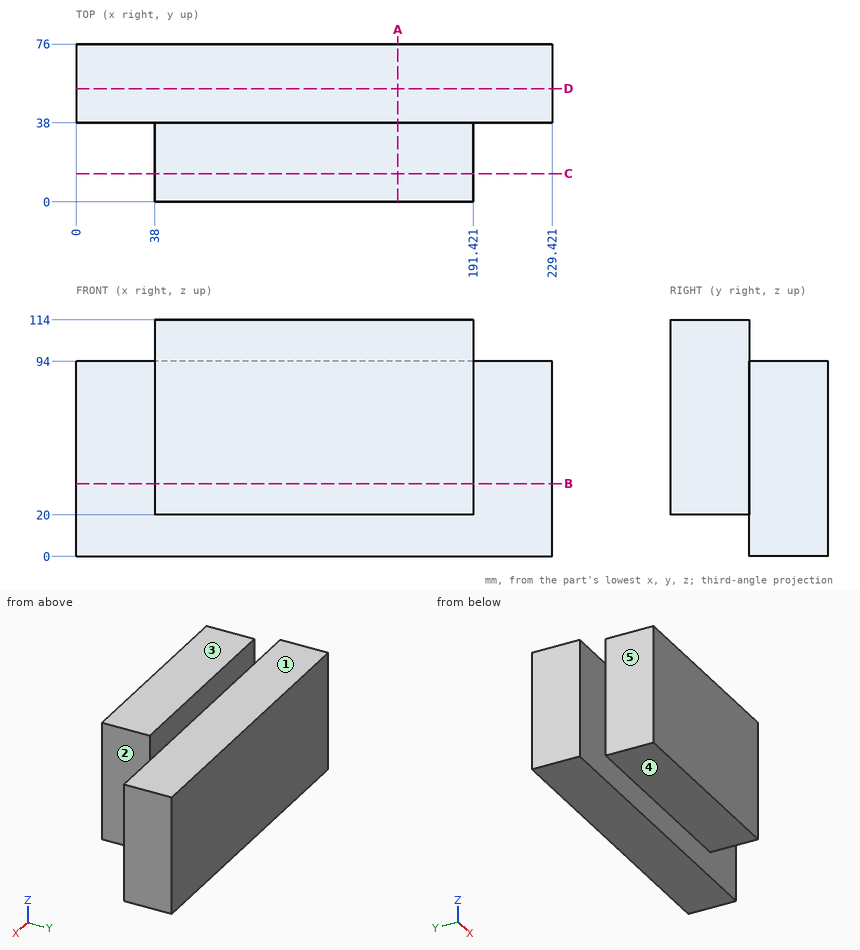
Geometry check sheet. Reference: drawing and pictorial views, mm from the part's lowest x, y, z. A direction names the side the tool comes from. Round coordinates to 2 decimals unless told otherwise and drop trailing zeros. Write each loop counter-clockwise with the first axis right and the second up, starting at its lowest first coordinate (ties: lowest second). Pieces come first, ordered by that corner, then holes.
1. Section check A-A on x = 155. Enter the section's corners in (y, z).
2. Access from +Z, -Z, +X, -X, +Y, -Y to the whole of each face (thin tool, end or side, straight path). Record for the marked faces 1, 2, 3, 4 and 5.
3. Gauge pin test, flat ends, axial feed: P1, Ø1.5, axis at x = 87.5, z = 95, coming from the +Y side; P2, Ø2, axis at x = 76.5, y = 15, coming from the -Z side; P3, Ø3, axis at y = 34.5, z = 57, coming from the -X side. Record the tip position at first contact, or that the pin passes through.
4. Section check C-C on y = 13.5. Enter the section's corners in (x, z), plus the area to 3 significant figures.
5. Scan lines: L1, parallel to X at y = 29, z = 50.5; L2, parallel to Z at x = 165, y = 42; L3, parallel to Y at x = 17, z = 79.5. Record each from-to range of solid material in increasing order.
6. Section check B-B on z = 35. Enter the section's corners in (x, y).
7. Section check D-D on y = 54.5. Enter the section's corners in (x, z), plus the area to 3 significant figures.
Answer:
1. outline: (0, 20) - (38, 20) - (38, 0) - (76, 0) - (76, 94) - (38, 94) - (38, 114) - (0, 114) - close
2. face 1: +Z, +X, -X, +Y
2. face 2: +Z, -Z, +X, -Y
2. face 3: +Z, +X, -X, +Y, -Y
2. face 4: -Z, +X, -X, -Y
2. face 5: +Z, -Z, -X, -Y
3. P1: stops at y = 38
3. P2: stops at z = 20
3. P3: stops at x = 38
4. outline: (38, 20) - (191.42, 20) - (191.42, 114) - (38, 114) - close
4. area: 14,400 mm2
5. L1: x = 38 to 191.42
5. L2: z = 0 to 94
5. L3: y = 38 to 76
6. outline: (0, 38) - (38, 38) - (38, 0) - (191.42, 0) - (191.42, 38) - (229.42, 38) - (229.42, 76) - (0, 76) - close
7. outline: (0, 0) - (229.42, 0) - (229.42, 94) - (0, 94) - close
7. area: 21,600 mm2
